Can you work these out from the drawing? Everything is in mm from the part's minimum corner. Round coordinates to 2 decimals unless told otherwise and drop trailing zeros. Write each loop counter-clockwise with the first axis right and the second up, starting at its lowest first coordinate (ties: lowest second). Pieces come first, ordered by that corner, then holes. Notation, with made-up numbers: (37.5, 22.5) -> (42.5, 22.5) arc R28 cw to (42.5, 56.5) -> close; hole circle Ø5 at (10, 48.25). An arc over 180 degrees is marked (long way). Answer as CSV lines item,"result". Start each with the question number.
Q1. Imagine slicing it at D-D on y = 4.75. Please give me the cut outline in (x, z).
Q2. Imagine slicing it at B-B on z = 16.5. Please give me the cut outline in (x, y).
Q3. If we mould it in two halves opening along X, with no side actions, what happens to the marked faces 1, 2 and 3? For each: pulls with the +X half, pulls with the -X half, needs draft (parallel to the pull), parting line crosses it, or undercut.
Q4. Imagine slicing it at C-C on y = 16.25. Please give me the cut outline in (x, z), and give its area (3 significant figures).
Q5. If I drill on line 1 (Z direction, x = 16.5, y = 12); line 2 (Z direction, x = 16.5, y = 3.05), over which ranges is the centre line in solid material (lowest first)? Write a range as [from, to].
Q6. Imagine slicing it at A-A on x = 16.5. Please give me the cut outline in (y, z), and give its area (3 significant figures).
Q7. Will these pins go through, and if not, where does the flat tip stop? pin 1 Ø2 at (x, y) = (20, 5.5) entering from -Z; pin 2 Ø2 at (x, z) = (23.5, 14) entering from +Y.
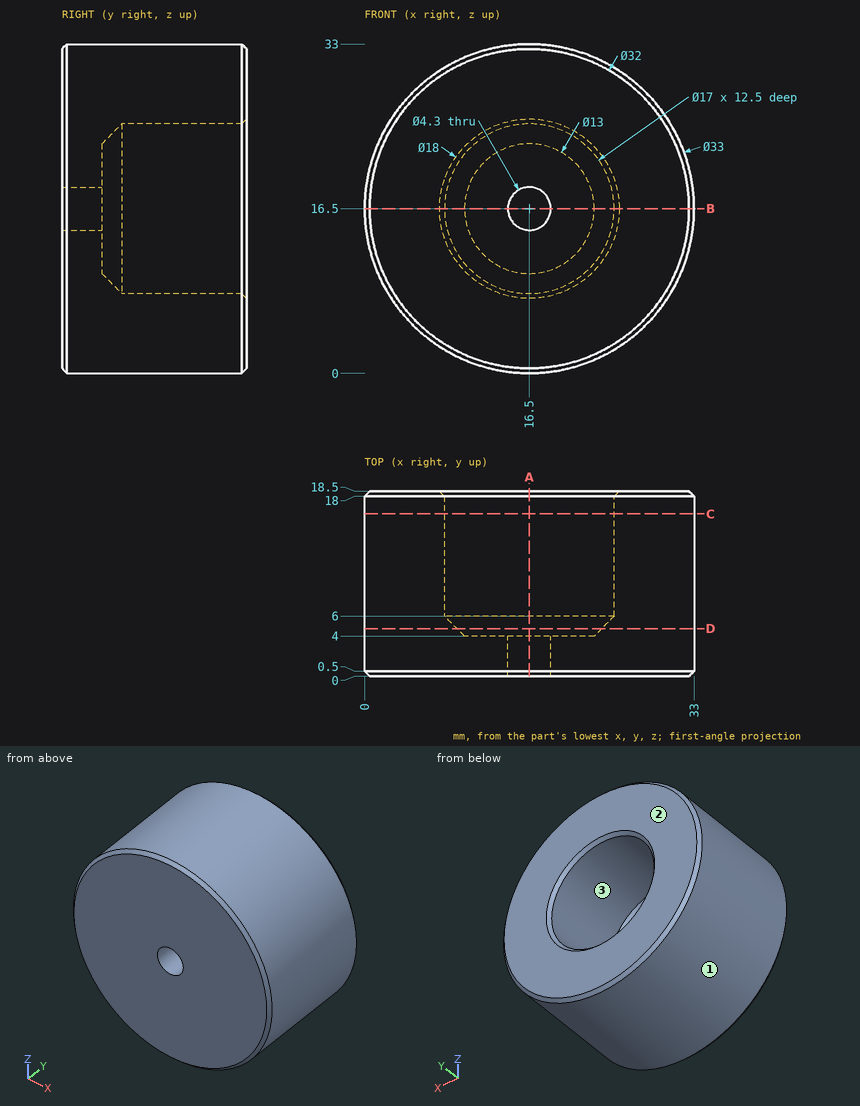
Checks:
1,outline,"circle Ø33 at (16.5, 16.5); hole circle Ø14.5 at (16.5, 16.5)"
2,outline,"(0, 0.5) -> (0.5, 0) -> (14.35, 0) -> (14.35, 4) -> (10, 4) -> (8, 6) -> (8, 18) -> (7.5, 18.5) -> (0.5, 18.5) -> (0, 18) -> close; (18.65, 0) -> (32.5, 0) -> (33, 0.5) -> (33, 18) -> (32.5, 18.5) -> (25.5, 18.5) -> (25, 18) -> (25, 6) -> (23, 4) -> (18.65, 4) -> close"
3,face 1,"parting line crosses it"
3,face 2,"needs draft"
3,face 3,"undercut"
4,outline,"circle Ø33 at (16.5, 16.5); hole circle Ø17 at (16.5, 16.5)"
4,area,"628 mm^2"
5,line 1,"[0, 8], [25, 33]"
5,line 2,"[0, 14.35], [18.65, 33]"
6,outline,"(0, 0.5) -> (0.5, 0) -> (18, 0) -> (18.5, 0.5) -> (18.5, 7.5) -> (18, 8) -> (6, 8) -> (4, 10) -> (4, 14.35) -> (0, 14.35) -> close; (0, 18.65) -> (4, 18.65) -> (4, 23) -> (6, 25) -> (18, 25) -> (18.5, 25.5) -> (18.5, 32.5) -> (18, 33) -> (0.5, 33) -> (0, 32.5) -> close"
6,area,"350 mm^2"
7,pin 1,"z = 0.19"
7,pin 2,"y = 5.93"
